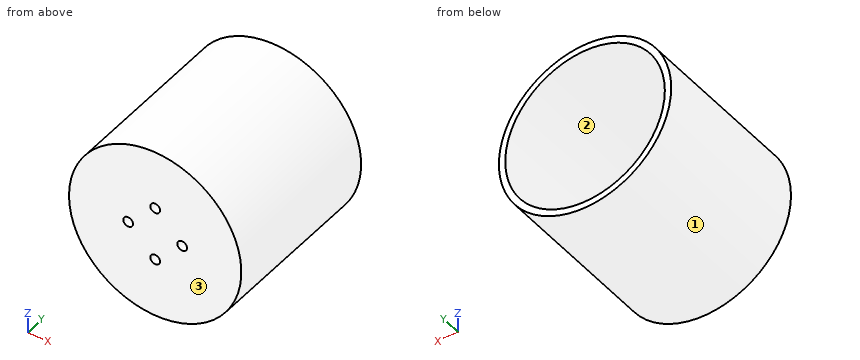
from build123d import *

# Parameters (mm, degrees)
SKETCH2_R                   = 2.3
CUT_EXTRUDE1_DEPTH          = 5.5
CUT_EXTRUDE1_DRAFT          = -4.35
CIRPATTERN1_COPY_1_SKETCH_R = 2.3
CIRPATTERN1_COPY_1_DEPTH    = 5.5
CIRPATTERN1_COPY_1_DRAFT    = -4.35
CIRPATTERN1_COPY_2_SKETCH_R = 2.3
CIRPATTERN1_COPY_2_DEPTH    = 5.5
CIRPATTERN1_COPY_2_DRAFT    = -4.35
CIRPATTERN1_COPY_3_SKETCH_R = 2.3
CIRPATTERN1_COPY_3_DEPTH    = 5.5
CIRPATTERN1_COPY_3_DRAFT    = -4.35


with BuildPart() as part:
    # Sketch1 → Revolve1 (revolve)
    with BuildSketch(Plane.XY):
        with BuildLine():
            Line((0, 0), (-40.5, 0))
            Line((-40.5, 0), (-40.5, 80))
            Line((-40.5, 80), (-37.5, 80))
            Line((-37.5, 80), (-37.5, 15.5))
            ThreePointArc((-37.5, 15.5), (-34.571067812, 8.428932188), (-27.5, 5.5))
            Line((-27.5, 5.5), (0, 5.5))
            Line((0, 5.5), (0, 0))
        make_face()
    revolve(axis=Axis((0, 5.5, 0), (0, -1, 0)))


with BuildPart() as cut_extrude1_tool:
    # Sketch2 → Cut-Extrude1 (with draft: the straight prism first)
    with BuildSketch(Plane.XZ):
        with Locations((0, 12.7)):
            Circle(SKETCH2_R)
    extrude(amount=-CUT_EXTRUDE1_DEPTH)
    # Cut-Extrude1: the draft: its side faces are tilted about the plane it starts from
    cut_extrude1_sides = [cut_extrude1_tool.faces().sort_by_distance(p)[0] for p in [
        (-2.3, 2.75, 12.7),
    ]]
    draft(cut_extrude1_sides, Plane.XZ, CUT_EXTRUDE1_DRAFT)


with BuildPart() as part_1:
    add(part.part)

    # Cut-Extrude1: cut by cut_extrude1_tool
    add(cut_extrude1_tool.part, mode=Mode.SUBTRACT)


with BuildPart() as cirpattern1_copy_1_tool:
    # CirPattern1 copy 1 sketch → CirPattern1 copy 1 (with draft: the straight prism first)
    with BuildSketch(Plane(origin=(0, 0, 0), x_dir=(0, 0, -1), z_dir=(0, -1, 0))):
        with Locations((0, 12.7)):
            Circle(CIRPATTERN1_COPY_1_SKETCH_R)
    extrude(amount=-CIRPATTERN1_COPY_1_DEPTH)
    # CirPattern1 copy 1: the draft: its side faces are tilted about the plane it starts from
    cirpattern1_copy_1_sides = [cirpattern1_copy_1_tool.faces().sort_by_distance(p)[0] for p in [
        (12.7, 2.75, 2.3),
    ]]
    draft(cirpattern1_copy_1_sides, Plane(origin=(0, 0, 0), x_dir=(0, 0, -1), z_dir=(0, -1, 0)), CIRPATTERN1_COPY_1_DRAFT)


with BuildPart() as part_2:
    add(part_1.part)

    # CirPattern1 copy 1: cut by cirpattern1_copy_1_tool
    add(cirpattern1_copy_1_tool.part, mode=Mode.SUBTRACT)


with BuildPart() as cirpattern1_copy_2_tool:
    # CirPattern1 copy 2 sketch → CirPattern1 copy 2 (with draft: the straight prism first)
    with BuildSketch(Plane(origin=(0, 0, 0), x_dir=(-1, 0, 0), z_dir=(0, -1, 0))):
        with Locations((0, 12.7)):
            Circle(CIRPATTERN1_COPY_2_SKETCH_R)
    extrude(amount=-CIRPATTERN1_COPY_2_DEPTH)
    # CirPattern1 copy 2: the draft: its side faces are tilted about the plane it starts from
    cirpattern1_copy_2_sides = [cirpattern1_copy_2_tool.faces().sort_by_distance(p)[0] for p in [
        (2.3, 2.75, -12.7),
    ]]
    draft(cirpattern1_copy_2_sides, Plane(origin=(0, 0, 0), x_dir=(-1, 0, 0), z_dir=(0, -1, 0)), CIRPATTERN1_COPY_2_DRAFT)


with BuildPart() as part_3:
    add(part_2.part)

    # CirPattern1 copy 2: cut by cirpattern1_copy_2_tool
    add(cirpattern1_copy_2_tool.part, mode=Mode.SUBTRACT)


with BuildPart() as cirpattern1_copy_3_tool:
    # CirPattern1 copy 3 sketch → CirPattern1 copy 3 (with draft: the straight prism first)
    with BuildSketch(Plane(origin=(0, 0, 0), x_dir=(0, 0, 1), z_dir=(0, -1, 0))):
        with Locations((0, 12.7)):
            Circle(CIRPATTERN1_COPY_3_SKETCH_R)
    extrude(amount=-CIRPATTERN1_COPY_3_DEPTH)
    # CirPattern1 copy 3: the draft: its side faces are tilted about the plane it starts from
    cirpattern1_copy_3_sides = [cirpattern1_copy_3_tool.faces().sort_by_distance(p)[0] for p in [
        (-12.7, 2.75, -2.3),
    ]]
    draft(cirpattern1_copy_3_sides, Plane(origin=(0, 0, 0), x_dir=(0, 0, 1), z_dir=(0, -1, 0)), CIRPATTERN1_COPY_3_DRAFT)


with BuildPart() as part_4:
    add(part_3.part)

    # CirPattern1 copy 3: cut by cirpattern1_copy_3_tool
    add(cirpattern1_copy_3_tool.part, mode=Mode.SUBTRACT)


solid = part_4.part
Design review of the part built by this model. Coordinates are the model's own, in mm. Face numbers are marked on the shaded views. Give positions to 0.01 mm unless a question says otherwise; leave off trailing zeros. Write each loop counter-clockwise with the first axis right and the second up, starting at its lowest first coordinate (ties: lowest second). Pieces come first, ordered by that corner, then holes. Notation, with made-up numbers: M -4,55 L 21,55 A21 ccw 21,62 Z; hole C 9.5,75.25 d1. An arc over 180 degrees is marked long. Return JSON: item names as keys, results as strings. Group by question number.
Item 1: Clearance check with flat-ended pins moving along their axes: pin 1 Ø5 at (x, y) = (-24.5, 39.5) entering from -Z; pin 2 Ø12 at (x, z) = (25.5, 14) entering from +Y; pin 3 Ø10 at (x, y) = (23, 8) entering from -Z; pin 4 Ø8 at (x, z) = (-19.5, -27.5) entering from +Y. State where each tip first meets the part, or that it passes through.
Item 2: Wall thickness on line 1 along Z through (x, y) = (0, 63); line 2 along Y through (x, z) = (20, -4.5): over which ranges is each line inside the solid? List them lowest first.
Item 3: The part is to be moulded in two halves that separate along X. For the marked faces 1, 2 and 3, say which applies: pulls with the +X half, pulls with the -X half, needs draft (parallel to the pull), parting line crosses it, or undercut.
Item 4: Take a section at A-A (y = 60). Give the boundary of the cut face in (x, z).
Return value:
{
 "1": {"pin 1": "stops at z = -34", "pin 2": "stops at y = 8.99", "pin 3": "stops at z = -36.28", "pin 4": "stops at y = 80"},
 "2": {"line 1": "z = -40.5 to -37.5, 37.5 to 40.5", "line 2": "y = 0 to 5.5"},
 "3": {"face 1": "parting line crosses it", "face 2": "undercut", "face 3": "needs draft"},
 "4": {"outline": "C 0,0 d81; hole C 0,0 d75"}
}
